Work out the finished part from the listing and answer in its coordinate system (mm). A direction names the side the tool comes from. Give positions to 0.01 mm unless a question says otherwise; leave off trailing zeros. Order: outer loops, then holes, each group sorted by start corner. A loop starts at its lowest first (then second) coordinate and runs counter-clockwise, first axis right, second up. Notation, with made-up numbers: M 83,47 L 101,47 A14 ccw 101,66 Z; hole C 3.25,14 d9. An arc over 180 degrees is marked long. One line per item, written item: value.
from build123d import *

# Parameters (mm, degrees)
F1_DEPTH = 33
F2_W     = 13
F2_H     = 22.75
F3_DEPTH = 11
F4_W     = 13
F4_H     = 3
F5_DEPTH = 5


# Not quite as in the source:
# - a feature of the source that left no trace in its solid (it failed there, or was rolled back) is left out


with BuildPart() as f1:
    # F0 (on Front) → F1 (new body)
    with BuildSketch(Plane.XZ):
        Polygon((-10.526334039, 27), (-29.5, 0), (-5, 0), (-5, 8.67), (5, 8.67), (5, 0), (28.947331922, 0), (9.973665961, 27), align=None)
    extrude(amount=F1_DEPTH)

    # F2 (on face) → F3 (cut)
    with BuildSketch(Plane.XZ.offset(33)):
        with Locations((0, 15.625)):
            Rectangle(F2_W, F2_H)
    extrude(amount=-F3_DEPTH, mode=Mode.SUBTRACT)

    # F4 (on face) → F5 (cut)
    with BuildSketch(Plane.XZ.offset(22)):
        with Locations((0, 23.5)):
            Rectangle(F4_W, F4_H)
    extrude(amount=-F5_DEPTH, mode=Mode.SUBTRACT)


solid = f1.part
(1) Given P1, Ø1, axis at x = -2, z = 26.5, coming from the -Y side; P2, Ø2.5, axis at y = -8.5, z = 6.5, coming from the +X side; P3, Ø3, axis at x = 0, y = -15, coming from the -Z side, each flat-ended and moving along its own axis, determine where each tip first touches the part or whether it passes through.
Findings:
P1: stops at y = -22
P2: stops at x = 25.26
P3: stops at z = 8.67
(2) Determine the mould class of faces 1 (the flat face through (-15, -33, 11)), 2 (the flat face through (0, -11, 8.67)), 3 (the flat face through (19.6, -16.3, 13.3)) for opening direction X: pulls with the +X half, pulls with the -X half, needs draft (parallel to the pull), parting line crosses it, or undercut.
Findings:
face 1: needs draft
face 2: undercut
face 3: pulls with the +X half
(3) Find the intervals of material crossed by probe 1 along Z at (x, y) = (0, -19.5); probe 2 along Y at (x, z) = (0.5, 14); probe 3 along X at (y, z) = (-25, 8), in increasing order. Write a range as from..to.
Findings:
probe 1: z = 8.67..22, 25..27
probe 2: y = -22..0
probe 3: x = -23.88..-6.5, 6.5..23.33
(4) Section C-C, the plane y = -6.5 is taken. Give the vertices of the cut face in (x, z), then the cut area to 3 significant figures.
Findings:
outline: M -29.5,0 L -5,0 L -5,8.67 L 5,8.67 L 5,0 L 28.95,0 L 9.97,27 L -10.53,27 Z
area: 979 mm^2
(5) Section B-B, the plane x = 2 is taken. Give the vertices of the cut face in (y, z).
Findings:
outline: M -22,8.67 L 0,8.67 L 0,27 L -22,27 L -22,25 L -17,25 L -17,22 L -22,22 Z
(6) Which of the six approach directions +Z, -Z, +X, -X, +Y, -Y give full straight-line access (tool end or side, diameter ignored) to faces 4 (the flat face through (0, -22, 15)), 5 (the flat face through (0, -20, 25)), 6 (the flat face through (-19.88, -16.27, 13.69)), 7 (the flat face through (-5, -13, 4)), 8 (the flat face through (-1, 0, 11))?
Findings:
face 4: +Z, -Y
face 5: -Y
face 6: +Z, -X, +Y, -Y
face 7: -Z, +Y, -Y
face 8: +Z, -Z, +X, -X, +Y
(7) Section A-A, the plane y = -26 is taken. Give the vertices of the cut face in (x, z), then the cut area to 3 significant figures.
Findings:
outline: M -29.5,0 L -5,0 L -5,4.25 L -6.5,4.25 L -6.5,27 L -10.53,27 Z; M 5,0 L 28.95,0 L 9.97,27 L 6.5,27 L 6.5,4.25 L 5,4.25 Z
area: 728 mm^2
(8) Section D-D, the plane z = 5 is taken. Give the vertices of the cut face in (x, y), then the cut area to 3 significant figures.
Findings:
outline: M -25.99,-33 L -6.5,-33 L -6.5,-22 L -5,-22 L -5,0 L -25.99,0 Z; M 5,-22 L 6.5,-22 L 6.5,-33 L 25.43,-33 L 25.43,0 L 5,0 Z
area: 1,330 mm^2
